Build history of the part. All positions in model axes, mm. A direction names the side the tool comes from. Give positions to 0.01 mm unless a question says otherwise; leave off trailing zeros. Loops run counter-clockwise (first coordinate to the right, second up) from the corner with the lowest first, then second, coordinate; pieces in that order, holes last. Notation, with made-up numbers: (30, 37.5) -> (80, 37.5) arc R31 cw to (80, 76.5) -> close; hole circle Ø3 at (83.25, 21). An arc over 180 degrees is marked (long way). Answer as a JSON object with one key per item and string values. Group by question number.
Q1. Tool access for faces 5 (the flat face through (1.32, 0.3, -13.9)), 6 (the flat face through (4.82, 0.3, -13.9)), 7 (the flat face through (3, 0.9, -2)), 8 (the flat face through (3, -13, -17.48)), 9 (the flat face through (3, -13, -1.74)): list every direction of +Z, -Z, +X, -X, +Y, -Y with a clear straight run to the whole face (end or side of a thin tool).
Q2. Two-plate mould, pull along Y, no slides. Class faces 1 (the cylindrical face through (3.03, -6.49, -15.65)), 2 (the flat face through (0, -5, -10)), 3 (the cylindrical face through (3.03, -6.31, -4.84)), 4 (the flat face through (3, 1.2, -2)): pulls with the +Y half, pulls with the -Y half, needs draft (parallel to the pull), parting line crosses it, or undercut.
Q3. Wall check: probe 1 along Y at (x, z) = (1.5, -5); probe 2 along Z at (x, y) = (1.5, -13.5); probe 3 along Y at (x, z) = (4.25, -0.5). Give the ranges that are in metal, low to high. Write a range as from..to.
Q4. Band-saw the part on D-D, the plane z = -15.5. Write the cut outline in (x, y), plus the area to 3 significant figures.
Q5. Band-saw the part on C-C, the plane x = 2.25. Write the cut outline in (y, z) (3 decimals).
Q6. Band-saw the part on B-B, the plane y = -12. Write the cut outline in (x, z), plus the area to 3 significant figures.
Q7. Band-saw the part on A-A, the plane z = -7. Write the cut outline in (x, y).
Q8. Drop flat-ended pins along their axis: pin 1 (2.5 mm diameter, centred on x = 3, y = -11.5, fed in from +Z); pin 2 (2 mm diameter, centred on x = 2, z = 3.5, fed in from -Y); pin 3 (1.6 mm diameter, centred on x = 3, y = -12, fed in from +Z); pin 4 (1.4 mm diameter, centred on y = -7.5, z = -5, fed in from +X). Give the stop position or say it passes through.
from build123d import *

# Parameters (mm, degrees)
SKETCH1_W           = 20
SKETCH1_H           = 10.5
SKETCH1_R           = 1.2
BOSS_EXTRUDE1_DEPTH = 6.14
BOSS_EXTRUDE2_DEPTH = 2
BOSS_EXTRUDE5_DEPTH = 1.75
SKETCH4_W           = 0.42
SKETCH4_H           = 4.5
BOSS_EXTRUDE6_DEPTH = 1.6


with BuildPart() as part:
    # Sketch1 → Boss-Extrude1 (new body)
    with BuildSketch(Plane(origin=(0, 0, 0), x_dir=(0, 0, -1), z_dir=(1, 0, 0))):
        with Locations((10, -5.25)):
            Rectangle(SKETCH1_W, SKETCH1_H)
        with Locations((5, -7.5)):
            Circle(SKETCH1_R, mode=Mode.SUBTRACT)
        with Locations((15, -7.5)):
            Circle(SKETCH1_R, mode=Mode.SUBTRACT)
    extrude(amount=BOSS_EXTRUDE1_DEPTH)

    # Sketch2 → Boss-Extrude2 (add, symmetric)
    with BuildSketch(Plane(origin=(3.07, 0, 0), x_dir=(0, 0, -1), z_dir=(1, 0, 0))):
        with BuildLine():
            Line((16.2, 0.9), (-12.6, 0.9))
            Line((-12.6, 0.9), (-12.6, 1.2))
            Line((-12.6, 1.2), (16.2, 1.2))
            ThreePointArc((16.2, 1.2), (17.048528137, 0.848528137), (17.4, 0))
            Line((17.4, 0), (17.1, 0))
            ThreePointArc((17.1, 0), (16.836396103, 0.636396103), (16.2, 0.9))
        make_face()
    extrude(amount=BOSS_EXTRUDE2_DEPTH, both=True)

    # Sketch3 → Boss-Extrude5 (add, symmetric)
    with BuildSketch(Plane(origin=(3.07, 0, 0), x_dir=(0, 0, -1), z_dir=(1, 0, 0))):
        with BuildLine():
            Line((13.025, 0), (14.775, 0))
            ThreePointArc((14.775, 0), (13.9, 0.875), (13.025, 0))
        make_face()
    extrude(amount=BOSS_EXTRUDE5_DEPTH, both=True)

    # Sketch4 → Boss-Extrude6 (add, symmetric)
    with BuildSketch(Plane(origin=(3.07, 0, 0), x_dir=(0, 0, -1), z_dir=(1, 0, 0))):
        with Locations((1.95, -12.75)):
            Rectangle(SKETCH4_W, SKETCH4_H)
        with Locations((9.23, -12.75)):
            Rectangle(SKETCH4_W, SKETCH4_H)
        with Locations((17.69, -12.75)):
            Rectangle(SKETCH4_W, SKETCH4_H)
    extrude(amount=BOSS_EXTRUDE6_DEPTH, both=True)


solid = part.part
Worked answers:
{
 "1": {"face 5": "+Z, -X", "face 6": "+Z, +X", "face 7": "+Z, +X, -X", "face 8": "+X, -X, -Y", "face 9": "+Z, +X, -X, -Y"},
 "2": {"face 1": "undercut", "face 2": "needs draft", "face 3": "undercut", "face 4": "pulls with the +Y half"},
 "3": {"probe 1": "-10.5..-8.7, -6.3..0, 0.9..1.2", "probe 2": "-17.9..-17.48, -9.44..-9.02, -2.16..-1.74", "probe 3": "-10.5..0, 0.9..1.2"},
 "4": {"outline": "(0, -10.5) -> (6.14, -10.5) -> (6.14, -8.59) -> (0, -8.59) -> close; (0, -6.41) -> (6.14, -6.41) -> (6.14, 0) -> (0, 0) -> close; (1.07, 0.9) -> (5.07, 0.9) -> (5.07, 1.2) -> (1.07, 1.2) -> close", "area": "52.3 mm2"},
 "5": {"outline": "(-15, -17.9) -> (-10.5, -17.9) -> (-10.5, -20) -> (0, -20) -> (0, -17.4) arc R1.2 ccw to (1.2, -16.2) -> (1.2, 12.6) -> (0.9, 12.6) -> (0.9, -16.2) arc R0.9 cw to (0, -17.1) -> (0, -14.775) arc R0.875 ccw to (0, -13.025) -> (0, 0) -> (-10.5, 0) -> (-10.5, -1.74) -> (-15, -1.74) -> (-15, -2.16) -> (-10.5, -2.16) -> (-10.5, -9.02) -> (-15, -9.02) -> (-15, -9.44) -> (-10.5, -9.44) -> (-10.5, -17.48) -> (-15, -17.48) -> close; hole circle Ø2.4 at (-7.5, -15); hole circle Ø2.4 at (-7.5, -5)"},
 "6": {"outline": "(1.47, -17.9) -> (4.67, -17.9) -> (4.67, -17.48) -> (1.47, -17.48) -> close; (1.47, -9.44) -> (4.67, -9.44) -> (4.67, -9.02) -> (1.47, -9.02) -> close; (1.47, -2.16) -> (4.67, -2.16) -> (4.67, -1.74) -> (1.47, -1.74) -> close", "area": "4.03 mm2"},
 "7": {"outline": "(0, -10.5) -> (6.14, -10.5) -> (6.14, 0) -> (0, 0) -> close; (1.07, 0.9) -> (5.07, 0.9) -> (5.07, 1.2) -> (1.07, 1.2) -> close"},
 "8": {"pin 1": "z = 0", "pin 2": "y = 0.9", "pin 3": "z = -1.74", "pin 4": "through"}
}
